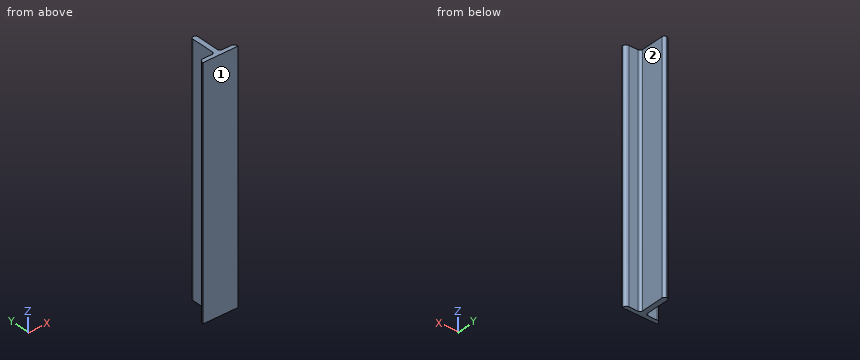
```python
from build123d import *

# Parameters (mm, degrees)
PAD_DEPTH = 150


with BuildPart() as part:
    # Sketch001 → Pad (new body)
    with BuildSketch(Plane.XY):
        with BuildLine():
            Line((-38.093584, -18.453745), (-32.287479, -18.453745))
            ThreePointArc((-32.287479, -18.453745), (-31.259526, -18.027953), (-30.833734, -17))
            Line((-30.833734, -17), (-30.833734, -2.438641))
            ThreePointArc((-29.37999, -0.984896), (-30.407943, -1.410688), (-30.833734, -2.438641))
            Line((-29.37999, -0.984896), (-29.155547, -0.984896))
            ThreePointArc((-27.701803, -2.438641), (-28.127595, -1.410688), (-29.155547, -0.984896))
            Line((-27.701803, -2.438641), (-27.701803, -17))
            ThreePointArc((-27.701803, -17), (-27.276011, -18.027953), (-26.248058, -18.453745))
            Line((-26.248058, -18.453745), (-20.441954, -18.453745))
            ThreePointArc((-18.368877, -20.526822), (-18.976067, -19.060935), (-20.441954, -18.453745))
            Line((-18.368877, -20.998255), (-18.368877, -20.526822))
            Line((-18.368877, -20.998255), (-40.16666, -20.998255))
            Line((-40.16666, -20.998255), (-40.16666, -20.526822))
            ThreePointArc((-38.093584, -18.453745), (-39.55947, -19.060935), (-40.16666, -20.526822))
        make_face()
    extrude(amount=PAD_DEPTH)


solid = part.part
```
The model under review builds one solid part; all positions refer to its coordinate system, in mm. Face numbers are marked on the shaded views. Round coordinates to 2 decimals unless told otherwise and drop trailing zeros. Order: outer loops, then holes, each group sorted by start corner. A loop starts at its lowest first (then second) coordinate and runs counter-clockwise, first axis right, second up.
(1) Wall thickness on L1, parallel to X at y = -13, z = 81.5; L2, parallel to Y at x = -24, z = 11; L3, parallel to X at y = -17.75, z = 42.5: over which ranges is each line inside the solid? List them lowest first.
Working result:
L1: x = -30.83 to -27.7
L2: y = -21 to -18.45
L3: x = -31.04 to -27.49
(2) Take a section at C-C, the plane y = -11.5. State the section outline as (x, z) points.
Working result:
outline: (-30.83, 0) - (-27.7, 0) - (-27.7, 150) - (-30.83, 150) - close
(3) Take a section at B-B, the plane x = -25. State the section outline as (y, z) points.
Working result:
outline: (-21, 0) - (-18.45, 0) - (-18.45, 150) - (-21, 150) - close
(4) Take a section at A-A, the plane z = 130.5. State the section outline as (x, y) points, plus the area to 3 significant figures.
Working result:
outline: (-40.17, -21) - (-18.37, -21) - (-18.37, -20.53) arc R2.07 ccw to (-20.44, -18.45) - (-26.25, -18.45) arc R1.45 cw to (-27.7, -17) - (-27.7, -2.44) arc R1.45 ccw to (-29.16, -0.98) - (-29.38, -0.98) arc R1.45 ccw to (-30.83, -2.44) - (-30.83, -17) arc R1.45 cw to (-32.29, -18.45) - (-38.09, -18.45) arc R2.07 ccw to (-40.17, -20.53) - close
area: 108 mm2
(5) Mouldability with a two-part tool opening along X and no side actions: class the marked faces 1 and 2 as released by +X, released by -X, zero draft, split by the parting line, or undercut.
Working result:
face 1: zero draft
face 2: released by +X
(6) For P1, Ø4.5, axis at x = -24.5, z = 81, coming from the +Y side; P2, Ø1.5, axis at x = -25, y = -7.5, coming from the +Z side; P3, Ø10, axis at y = -11.5, z = 73.5, coming from the +X side; P4, Ø1, axis at x = -37.5, z = 38.5, coming from the +Y side, all flat-tipped, find the tip position at first contact; note any pin that passes through.
Working result:
P1: stops at y = -18.36
P2: passes through
P3: stops at x = -27.7
P4: stops at y = -18.45
